Model file for the job. Use its own axes, mm. Face numbers are marked on the shaded views. Round coordinates to 2 decimals unless told otherwise and drop trailing zeros. Order: outer loops, then holes, each group sorted by start corner. A loop starts at its lowest first (then second) coordinate and runs counter-clockwise, first axis right, second up. Notation, with made-up numbers: (-11.5, 71.5) -> (30.5, 71.5) arc R20 cw to (30.5, 86.5) -> close; hole circle Ø10 at (12, 49). An arc over 180 degrees is marked (long way). Answer as CSV lines item,"result".
```python
from build123d import *

# Parameters (mm, degrees)
F0_R     = 190.5
F1_DEPTH = 12.7
F2_R     = 12.7
F2_R_2   = 1.8096717608
F3_DEPTH = 685.8
F4_R     = 190.5
F5_DEPTH = 12.7
F6_R     = 5.08


with BuildPart() as f1:
    # F0 (on Front) → F1 (new body)
    with BuildSketch(Plane.XZ):
        with Locations((-12.7692446113, 10.287723504)):
            Circle(F0_R)
    extrude(amount=F1_DEPTH)

    # F2 (on face) → F3 (join)
    with BuildSketch(Plane.XZ.offset(12.7)):
        with Locations((-12.7692446113, 10.287723504)):
            Circle(F2_R)
        with Locations((-12.7692446113, 10.287723504)):
            Circle(F2_R_2, mode=Mode.SUBTRACT)
    extrude(amount=F3_DEPTH)

    # F4 (on face) → F5 (join)
    with BuildSketch(Plane.XZ.offset(698.5)):
        with Locations((-12.7692446113, 10.287723504)):
            Circle(F4_R)
    extrude(amount=F5_DEPTH)

    # F6
    f6_edges = [f1.edges().sort_by_distance(p)[0] for p in [
        (-203.269245, -711.2, 10.287724),
        (-203.269245, -698.5, 10.287724),
        (-203.269245, -12.7, 10.287724),
        (-203.269245, 0, 10.287724),
    ]]
    fillet(f6_edges, radius=F6_R)


solid = f1.part
```
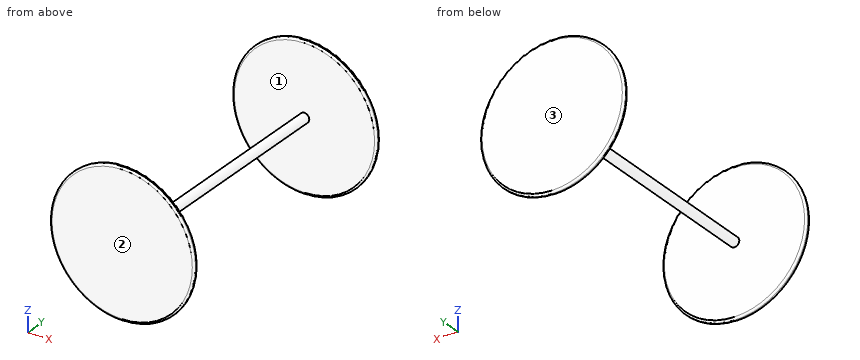
Q1. Saw through at A-A (y = -63.5). Write the cut outline in (x, z).
Checks:
outline,"circle Ø25.4 at (-12.77, 10.29); hole circle Ø3.62 at (-12.77, 10.29)"
Q2. Wall check: L1, parallel to Y at x = -104, z = 54.5; L2, parallel to Z at x = -3, y = -653. Give the ranges that are in metal, low to high. Write a range as [from, to].
Checks:
L1,"[-711.2, -698.5], [-12.7, 0]"
L2,"[2.17, 18.4]"
Q3. Mould opens along Y. For the marked faces 1, 2 and 3 say: +Y half, -Y half, draft (parallel to the pull), parting line (faces both ways), or undercut.
Checks:
face 1,"undercut"
face 2,"-Y half"
face 3,"+Y half"
Q4. Flat gauge pin, fed straight in: pin 1 (1.5 mm diameter, centred on x = -4.5, y = -480.5, fed in from +Z). Where does the tip first touch, or does it go through?
Checks:
pin 1,"z = 20.52"
